from build123d import *

# Parameters (mm, degrees)
SKETCH1_W                = 50
SKETCH1_H                = 50
BOSS_EXTRUDE1_DEPTH      = 75
FILLET1_R                = 5
SKETCH2_W                = 42.5
SKETCH2_H                = 42.5
CUT_EXTRUDE1_DEPTH       = 70
FILLET2_R                = 3
SKETCH3_W                = 25.5
SKETCH3_H                = 3.75
SKETCH3_W_2              = 3.75
SKETCH3_H_2              = 25.5
CUT_EXTRUDE2_DEPTH       = 50
SKETCH4_W                = 20
SKETCH4_H                = 3.75
CUT_EXTRUDE3_DEPTH       = 70
SKETCH8_R                = 1.55
CUT_EXTRUDE5_DEPTH       = 5
SKETCH9_R                = 4
CUT_EXTRUDE6_DEPTH       = 5
MIRROR2_COPY_1_SKETCH_R  = 1.55
MIRROR2_COPY_1_DEPTH     = 5
MIRROR2_COPY_2_SKETCH_R  = 4
MIRROR2_COPY_2_DEPTH     = 5
BOSS_EXTRUDE2_DEPTH      = 25
BOSS_EXTRUDE2_DEPTH_BACK = 120
CUT_EXTRUDE8_DEPTH       = 15
SKETCH12_R               = 1.55
CUT_EXTRUDE9_DEPTH       = 15
SKETCH13_W               = 10
SKETCH13_H               = 42
BOSS_EXTRUDE3_DEPTH      = 15
BOSS_EXTRUDE3_DEPTH_BACK = 15
BOSS_EXTRUDE4_DEPTH      = 42
SKETCH16_W               = 30
SKETCH16_H               = 9
CUT_EXTRUDE10_DEPTH      = 10
SKETCH17_W               = 0.2
SKETCH17_H               = 42
CUT_EXTRUDE11_DEPTH      = 15
SKETCH18_W               = 24
SKETCH18_H               = 20
BOSS_EXTRUDE7_DEPTH      = 80
BOSS_EXTRUDE7_DEPTH_BACK = 3.75
SKETCH19_W               = 15
SKETCH19_H               = 16
CUT_EXTRUDE12_DEPTH      = 84


with BuildPart() as part:
    # Sketch1 → Boss-Extrude1 (new body)
    with BuildSketch(Plane(origin=(0, 0, 0), x_dir=(0, 0, -1), z_dir=(1, 0, 0))):
        Rectangle(SKETCH1_W, SKETCH1_H)
    extrude(amount=-BOSS_EXTRUDE1_DEPTH)

    # Fillet1
    fillet1_edges = [part.edges().sort_by_distance(p)[0] for p in [
        (-37.5, -25, -25),
        (-37.5, -25, 25),
        (-37.5, 25, 25),
        (-37.5, 25, -25),
    ]]
    fillet(fillet1_edges, radius=FILLET1_R)

    # Sketch2 → Cut-Extrude1 (cut)
    with BuildSketch(Plane(origin=(0, 0, 0), x_dir=(0, 0, -1), z_dir=(1, 0, 0))):
        Rectangle(SKETCH2_W, SKETCH2_H)
    extrude(amount=-CUT_EXTRUDE1_DEPTH, mode=Mode.SUBTRACT)

    # Fillet2
    fillet2_edges = [part.edges().sort_by_distance(p)[0] for p in [
        (-35, 21.25, -21.25),
        (-35, -21.25, -21.25),
        (-35, -21.25, 21.25),
        (-35, 21.25, 21.25),
    ]]
    fillet(fillet2_edges, radius=FILLET2_R)

    # Sketch3 → Cut-Extrude2 (cut)
    with BuildSketch(Plane(origin=(0, 0, 0), x_dir=(0, 0, -1), z_dir=(1, 0, 0))):
        with Locations((0, 23.125)):
            Rectangle(SKETCH3_W, SKETCH3_H)
        with Locations((-23.125, 0)):
            Rectangle(SKETCH3_W_2, SKETCH3_H_2)
        with Locations((23.125, 0)):
            Rectangle(SKETCH3_W_2, SKETCH3_H_2)
    extrude(amount=-CUT_EXTRUDE2_DEPTH, mode=Mode.SUBTRACT)

    # Sketch4 → Cut-Extrude3 (cut)
    with BuildSketch(Plane(origin=(0, 0, 0), x_dir=(0, 0, -1), z_dir=(1, 0, 0))):
        with Locations((0, -23.125)):
            Rectangle(SKETCH4_W, SKETCH4_H)
    extrude(amount=-CUT_EXTRUDE3_DEPTH, mode=Mode.SUBTRACT)

    # Sketch8 → Cut-Extrude5 (cut)
    with BuildSketch(Plane(origin=(0, 0, 0), x_dir=(0, 0, -1), z_dir=(1, 0, 0))):
        with Locations((-22, 21.6)):
            Circle(SKETCH8_R)
    cut_extrude5 = extrude(amount=-CUT_EXTRUDE5_DEPTH, mode=Mode.SUBTRACT)

    # Sketch9 → Cut-Extrude6 (cut)
    with BuildSketch(Plane(origin=(-5, 0, 0), x_dir=(0, 0, -1), z_dir=(1, 0, 0))):
        with Locations((-22, 21.6)):
            Circle(SKETCH9_R)
    cut_extrude6 = extrude(amount=-CUT_EXTRUDE6_DEPTH, mode=Mode.SUBTRACT)

    # Mirror1: Cut-Extrude5, Cut-Extrude6 across plane
    add(cut_extrude5.mirror(Plane.ZX), mode=Mode.SUBTRACT)
    add(cut_extrude6.mirror(Plane.ZX), mode=Mode.SUBTRACT)

    # Mirror2: Cut-Extrude5, Cut-Extrude6 across plane
    add(cut_extrude5.mirror(Plane.XY), mode=Mode.SUBTRACT)
    add(cut_extrude6.mirror(Plane.XY), mode=Mode.SUBTRACT)

    # Mirror2 copy 1 sketch → Mirror2 copy 1 (cut)
    with BuildSketch(Plane(origin=(0, 0, 0), x_dir=(0, 0, 1), z_dir=(1, 0, 0))):
        with Locations((-22, 21.6)):
            Circle(MIRROR2_COPY_1_SKETCH_R)
    extrude(amount=-MIRROR2_COPY_1_DEPTH, mode=Mode.SUBTRACT)

    # Mirror2 copy 2 sketch → Mirror2 copy 2 (cut)
    with BuildSketch(Plane(origin=(-5, 0, 0), x_dir=(0, 0, 1), z_dir=(1, 0, 0))):
        with Locations((-22, 21.6)):
            Circle(MIRROR2_COPY_2_SKETCH_R)
    extrude(amount=-MIRROR2_COPY_2_DEPTH, mode=Mode.SUBTRACT)

    # Sketch10 → Boss-Extrude2 (add, two sides)
    with BuildSketch(Plane(origin=(0, 0, 0), x_dir=(1, 0, 0), z_dir=(0, 1, 0))) as boss_extrude2_sk:
        with BuildLine():
            Line((-75, -21), (-75, 21))
            ThreePointArc((-75, 21), (-96, 0), (-75, -21))
        make_face()
    extrude(amount=BOSS_EXTRUDE2_DEPTH)
    extrude(boss_extrude2_sk.sketch, amount=-BOSS_EXTRUDE2_DEPTH_BACK)

    # Sketch11 → Cut-Extrude8 (cut)
    with BuildSketch(Plane.XZ.offset(120)):
        with BuildLine():
            Line((-85, 18.466185313), (-85, -18.466185313))
            ThreePointArc((-85, -18.466185313), (-80.158008745, -20.356692899), (-75, -21))
            Line((-75, -21), (-75, 21))
            ThreePointArc((-75, 21), (-80.158008745, 20.356692899), (-85, 18.466185313))
        make_face()
    extrude(amount=-CUT_EXTRUDE8_DEPTH, mode=Mode.SUBTRACT)

    # Sketch12 → Cut-Extrude9 (cut)
    with BuildSketch(Plane(origin=(-85, 0, 0), x_dir=(0, 0, -1), z_dir=(1, 0, 0))):
        with Locations((0, -112.5)):
            Circle(SKETCH12_R)
        with Locations((-6.5, -112.5)):
            Circle(SKETCH12_R)
        with Locations((6.5, -112.5)):
            Circle(SKETCH12_R)
    extrude(amount=-CUT_EXTRUDE9_DEPTH, mode=Mode.SUBTRACT)



with BuildPart() as body_2:
    # Sketch13 → Boss-Extrude3 (new body, two sides)
    with BuildSketch(Plane.XZ.offset(105)) as boss_extrude3_sk:
        with Locations((-70, 0)):
            Rectangle(SKETCH13_W, SKETCH13_H)
    extrude(amount=BOSS_EXTRUDE3_DEPTH)
    extrude(boss_extrude3_sk.sketch, amount=-BOSS_EXTRUDE3_DEPTH_BACK)


with BuildPart() as part_1:
    add(part.part)

    add(body_2.part)  # Boss-Extrude4 merges body 2
    # Sketch15 → Boss-Extrude4 (add)
    with BuildSketch(Plane.XY.offset(21)):
        Polygon((-65, -90), (-75, -90), (-75, -80), align=None)
    extrude(amount=-BOSS_EXTRUDE4_DEPTH)

    # Sketch16 → Cut-Extrude10 (cut)
    with BuildSketch(Plane(origin=(-65, 0, 0), x_dir=(0, 0, -1), z_dir=(1, 0, 0))):
        with Locations((0, -112.5)):
            Rectangle(SKETCH16_W, SKETCH16_H)
    extrude(amount=-CUT_EXTRUDE10_DEPTH, mode=Mode.SUBTRACT)

    # Sketch17 → Cut-Extrude11 (cut)
    with BuildSketch(Plane.XZ.offset(120)):
        with Locations((-74.9, 0)):
            Rectangle(SKETCH17_W, SKETCH17_H)
    extrude(amount=-CUT_EXTRUDE11_DEPTH, mode=Mode.SUBTRACT)

    # Sketch18 → Boss-Extrude7 (add, two sides)
    with BuildSketch(Plane.XZ.offset(25)) as boss_extrude7_sk:
        with Locations((-63, 0)):
            Rectangle(SKETCH18_W, SKETCH18_H)
    extrude(amount=BOSS_EXTRUDE7_DEPTH)
    extrude(boss_extrude7_sk.sketch, amount=-BOSS_EXTRUDE7_DEPTH_BACK)

    # Sketch19 → Cut-Extrude12 (cut)
    with BuildSketch(Plane(origin=(0, -21.25, 0), x_dir=(1, 0, 0), z_dir=(0, 1, 0))):
        with Locations((-62.5, 0)):
            Rectangle(SKETCH19_W, SKETCH19_H)
    extrude(amount=-CUT_EXTRUDE12_DEPTH, mode=Mode.SUBTRACT)


solid = part_1.part
Read the model definition and answer for the solid it produces. Units are mm, in the model's axes. A direction names the side the tool comes from. Round coordinates to 2 decimals unless told otherwise and drop trailing zeros. Write each loop counter-clockwise with the first axis right and the second up, starting at its lowest first coordinate (ties: lowest second). Pieces come first, ordered by that corner, then holes. Notation, with made-up numbers: M 11.5,22.25 L 26.5,22.25 A16 cw 26.5,48.25 Z; hole C 7,-29.75 d6. An arc over 180 degrees is marked long. Use a Markdown table: item, result.
1) Flat-ended cylindrical pins translate along their axes: pin 1 (2 mm diameter, centred on y = -40, z = -9.5, fed in from +X); pin 2 (4 mm diameter, centred on y = -1, z = -23, fed in from +X); pin 3 (1.1 mm diameter, centred on x = -17, y = -23, fed in from +Z). Find the tip coordinate at first contact, or state that the pin passes through.
Answers follow:
| item | result |
|---|---|
| pin 1 | stops at x = -51 |
| pin 2 | stops at x = -50 |
| pin 3 | stops at z = 24.36 |
2) The part is cut by section A-A (z = 0). Write down the section's boundary in (x, y).
Answers follow:
| item | result |
|---|---|
| outline | M -96,-120 L -85,-120 L -85,-114.05 L -96,-114.05 Z; M -96,-110.95 L -85,-110.95 L -85,-105 L -74.8,-105 L -74.8,-108 L -65,-108 L -65,-105.25 L -70,-105.25 L -70,21.25 L -50,21.25 L -50,25 L -96,25 Z; M -74.8,-120 L -65,-120 L -65,-117 L -74.8,-117 Z; M -55,-105 L -51,-105 L -51,-21.25 L -55,-21.25 Z |
3) A tool of negligible diameter and unlimited length cuts with its end or side. For faces 5 (the flat face through (-75, 0, 23)), 6 (the cylindrical face through (-7.465, 17.825, -23.323)), 7 (the flat face through (-75, -52, 16)), from which of +Z, -Z, +X, -X, +Y, -Y can it reach the whole face along a straight path? Write none if from no direction.
Answers follow:
| item | result |
|---|---|
| face 5 | +Z, -X, +Y, -Y |
| face 6 | +Y |
| face 7 | +Z, +X |
4) The part is cut by section C-C (y = -6). Write down the section's boundary in (x, z), plus the area to 3 significant figures.
Answers follow:
| item | result |
|---|---|
| outline | M -75,-25 L -50,-25 L -50,-21.25 L -70,-21.25 L -70,21.25 L -50,21.25 L -50,25 L -75,25 L -75,21 A21 ccw -75,-21 Z |
| area | 1,090 mm2 |
5) The part is cut by section B-B (x = -23). Give the number of separate pieces and of enclosed holes in the cut face, plus the area to 3 significant figures.
Answers follow:
| item | result |
|---|---|
| separate pieces | 4 |
| enclosed holes | 0 |
| area | 318 mm2 |
6) For a pull along Z with two mould halves and no side action, classify faces 1 (the flat face through (-70, -27, 0)), 2 (the flat face through (-65, -105.2, 9)), 3 (the flat face through (-63, -64, 10)), 4 (the cylindrical face through (-96, -46, 0)) as pulls with the +Z half, pulls with the -Z half, needs draft (parallel to the pull), parting line crosses it, or undercut.
Answers follow:
| item | result |
|---|---|
| face 1 | undercut |
| face 2 | needs draft |
| face 3 | pulls with the +Z half |
| face 4 | parting line crosses it |
7) Straight lines are drawn through the part: line 1 along Y through (x, z) = (-88, 6.5); line 2 along Z through (x, y) = (-93, -112); line 3 along Z through (x, y) = (-90.25, -112.5). For each, find the intervals that lie inside material, in ascending order. Write a range as [from, to].
Answers follow:
| item | result |
|---|---|
| line 1 | y = [-120, -114.05], [-110.95, 25] |
| line 2 | z = [-10.82, -7.97], [-5.03, -1.47], [1.47, 5.03], [7.97, 10.82] |
| line 3 | z = [-14.44, -8.05], [-4.95, -1.55], [1.55, 4.95], [8.05, 14.44] |
